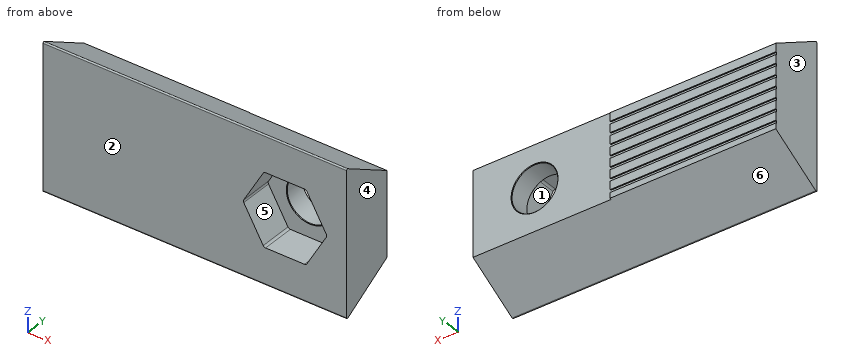
from build123d import *

# Parameters (mm, degrees)
SKETCH1_R                       = 4.15
BOSS_EXTRUDE1_DEPTH             = 10
CUT_EXTRUDE2_DEPTH              = 42.907636536
CUT_EXTRUDE2_DEPTH_BACK         = 42.907636536
SKETCH2_W                       = 0.5
SKETCH2_H                       = 0.2
BOSS_EXTRUDE2_REACH             = 43.908
BOSS_EXTRUDE2_DIRECTION_2_REACH = 43.908
SKETCH10_W                      = 15.230940108
SKETCH10_H                      = 0.2
CUT_EXTRUDE6_DEPTH              = 25
CUT_EXTRUDE5_DEPTH              = 6
FILLET3_R                       = 0.5
CHAMFER1_SIZE                   = 0.1


with BuildPart() as part:
    # Sketch1 → Boss-Extrude1 (new body)
    with BuildSketch(Plane(origin=(0, 0, 0), x_dir=(1, 0, 0), z_dir=(0, 1, 0))):
        Polygon((-15, -7.5), (15, -7.5), (40, -7.5), (40, 7.5), (15, 7.5), (-15, 7.5), align=None)
        with Locations(Location((28.85, 0, 0), (0, 0, 270))):
            Circle(SKETCH1_R, mode=Mode.SUBTRACT)
    extrude(amount=BOSS_EXTRUDE1_DEPTH)

    # Sketch2 → Cut-Extrude2 (cut, two sides: drawn at the far end of the back side and taken through both)
    with BuildSketch(Plane(origin=(0, 0, 0), x_dir=(0, 0, -1), z_dir=(1, 0, 0)).offset(-CUT_EXTRUDE2_DEPTH_BACK)):
        with Locations((-5.75, 9.9)):
            Rectangle(SKETCH2_W, SKETCH2_H)
        with Locations((-3.75, 9.9)):
            Rectangle(SKETCH2_W, SKETCH2_H)
        with Locations((-1.75, 9.9)):
            Rectangle(SKETCH2_W, SKETCH2_H)
        with Locations((0.25, 9.9)):
            Rectangle(SKETCH2_W, SKETCH2_H)
        with Locations((2.25, 9.9)):
            Rectangle(SKETCH2_W, SKETCH2_H)
        with Locations((4.25, 9.9)):
            Rectangle(SKETCH2_W, SKETCH2_H)
        with Locations((6.25, 9.9)):
            Rectangle(SKETCH2_W, SKETCH2_H)
    extrude(amount=CUT_EXTRUDE2_DEPTH + CUT_EXTRUDE2_DEPTH_BACK, mode=Mode.SUBTRACT)

    # Boss-Extrude2: up to this face of the body (flat: up to its plane)
    boss_extrude2_end = Plane(part.part.faces().sort_by_distance((40, 4.977026122, 0.001172137))[0])
    # Sketch3 → Boss-Extrude2 (add, up to the picked face)
    with BuildSketch(Plane(origin=(0, 0, 0), x_dir=(0, 0, -1), z_dir=(1, 0, 0)), mode=Mode.PRIVATE) as boss_extrude2_sk1:
        with BuildLine():
            Line((7.5, 10), (13.097822121, 0.304287674))
            ThreePointArc((13.097822121, 0.304287674), (13.097822121, 0.101429225), (12.92214155, 0))
            Line((12.92214155, 0), (7.5, 0))
            Line((7.5, 0), (7.5, 10))
        make_face()
    boss_extrude2_tool1 = split(extrude(boss_extrude2_sk1.sketch, amount=BOSS_EXTRUDE2_REACH, mode=Mode.PRIVATE), bisect_by=boss_extrude2_end, keep=Keep.BOTH, mode=Mode.PRIVATE)
    # Sketch3 → Boss-Extrude2 (add, up to the picked face)
    with BuildSketch(Plane(origin=(0, 0, 0), x_dir=(0, 0, -1), z_dir=(1, 0, 0)), mode=Mode.PRIVATE) as boss_extrude2_sk2:
        with BuildLine():
            Line((-7.5, 0), (-7.5, 10))
            Line((-7.5, 10), (-13.097822121, 0.304287674))
            ThreePointArc((-13.097822121, 0.304287674), (-13.097822121, 0.101429225), (-12.92214155, 0))
            Line((-12.92214155, 0), (-7.5, 0))
        make_face()
    boss_extrude2_tool2 = split(extrude(boss_extrude2_sk2.sketch, amount=BOSS_EXTRUDE2_REACH, mode=Mode.PRIVATE), bisect_by=boss_extrude2_end, keep=Keep.BOTH, mode=Mode.PRIVATE)
    add(boss_extrude2_tool1.solids().sort_by(Axis((0, 3.336518, -9.420866), (1, 0, 0)))[0])
    add(boss_extrude2_tool2.solids().sort_by(Axis((0, 3.336518, 9.420866), (1, 0, 0)))[0])

    # Boss-Extrude2 direction 2: up to this face of the body (flat: up to its plane)
    boss_extrude2_direction_2_end = Plane(part.part.faces().sort_by_distance((-15, 4.977026122, 0.001172137))[0])
    # Sketch3 → Boss-Extrude2 direction 2 (add, up to the picked face)
    with BuildSketch(Plane(origin=(0, 0, 0), x_dir=(0, 0, -1), z_dir=(1, 0, 0)), mode=Mode.PRIVATE) as boss_extrude2_direction_2_sk1:
        with BuildLine():
            Line((7.5, 10), (13.097822121, 0.304287674))
            ThreePointArc((13.097822121, 0.304287674), (13.097822121, 0.101429225), (12.92214155, 0))
            Line((12.92214155, 0), (7.5, 0))
            Line((7.5, 0), (7.5, 10))
        make_face()
    boss_extrude2_direction_2_tool1 = split(extrude(boss_extrude2_direction_2_sk1.sketch, amount=-BOSS_EXTRUDE2_DIRECTION_2_REACH, mode=Mode.PRIVATE), bisect_by=boss_extrude2_direction_2_end, keep=Keep.BOTH, mode=Mode.PRIVATE)
    # Sketch3 → Boss-Extrude2 direction 2 (add, up to the picked face)
    with BuildSketch(Plane(origin=(0, 0, 0), x_dir=(0, 0, -1), z_dir=(1, 0, 0)), mode=Mode.PRIVATE) as boss_extrude2_direction_2_sk2:
        with BuildLine():
            Line((-7.5, 0), (-7.5, 10))
            Line((-7.5, 10), (-13.097822121, 0.304287674))
            ThreePointArc((-13.097822121, 0.304287674), (-13.097822121, 0.101429225), (-12.92214155, 0))
            Line((-12.92214155, 0), (-7.5, 0))
        make_face()
    boss_extrude2_direction_2_tool2 = split(extrude(boss_extrude2_direction_2_sk2.sketch, amount=-BOSS_EXTRUDE2_DIRECTION_2_REACH, mode=Mode.PRIVATE), bisect_by=boss_extrude2_direction_2_end, keep=Keep.BOTH, mode=Mode.PRIVATE)
    add(boss_extrude2_direction_2_tool1.solids().sort_by(Axis((0, 3.336518, -9.420866), (-1, 0, 0)))[0])
    add(boss_extrude2_direction_2_tool2.solids().sort_by(Axis((0, 3.336518, 9.420866), (-1, 0, 0)))[0])

    # Sketch10 → Cut-Extrude6 (cut)
    with BuildSketch(Plane(origin=(40, 0, 0), x_dir=(0, 0, -1), z_dir=(1, 0, 0))):
        with Locations((0, 9.9)):
            Rectangle(SKETCH10_W, SKETCH10_H)
    extrude(amount=-CUT_EXTRUDE6_DEPTH, mode=Mode.SUBTRACT)

    # Sketch8 → Cut-Extrude5 (cut)
    with BuildSketch(Plane.XZ):
        Polygon((25.039488223, -6.6), (32.660511777, -6.6), (36.471023553, 0), (32.660511777, 6.6), (25.039488223, 6.6), (21.228976447, 0), align=None)
    extrude(amount=-CUT_EXTRUDE5_DEPTH, mode=Mode.SUBTRACT)

    # Fillet3
    fillet3_edges = [part.edges().sort_by_distance(p)[0] for p in [
        (25.039488223, 3, -6.6),
        (21.228976447, 3, 0),
        (25.039488223, 3, 6.6),
        (32.660511777, 3, 6.6),
        (36.471023553, 3, 0),
        (32.660511777, 3, -6.6),
    ]]
    fillet(fillet3_edges, radius=FILLET3_R)

    # Chamfer1
    chamfer1_edges = [part.edges().sort_by_distance(p)[0] for p in [
        (28.85, 9.8, -4.15),
        (28.85, 6, -4.15),
    ]]
    chamfer(chamfer1_edges, length=CHAMFER1_SIZE)


solid = part.part
Work out the finished part from the listing and answer in its coordinate system (mm). Face numbers are marked on the shaded views. A direction names the side the tool comes from. Round coordinates to 2 decimals unless told otherwise and drop trailing zeros. Write each loop counter-clockwise with the first axis right and the second up, starting at its lowest first coordinate (ties: lowest second). Pieces come first, ordered by that corner, then holes.
1) Given pin 1 Ø5 at (x, y) = (26.5, 4) entering from -Z; pin 2 Ø2 at (x, y) = (-8.5, 4.5) entering from +Z; pin 3 Ø2 at (x, y) = (0.5, 3) entering from +Z, each flat-ended and moving along its own axis, determine where each tip first touches the part or whether it passes through.
2) Straight lines are drawn through the part: line 1 (X direction, y = 7.05, z = 0); line 2 (Z direction, x = 28.85, y = 7.35); line 3 (Z direction, x = 28.85, y = 8). For each, find the intervals that lie inside material, in ascending order.
3) A tool of negligible diameter and unlimited length cuts with its end or side. For the marked faces 5 and 6, from which of +Z, -Z, +X, -X, +Y, -Y can it reach the whole face along a straight path? Write none if from no direction.
4) A cutting plane is placed at D-D (z = 9.5). Give the vertices of the cut face in (x, y).
5) A cutting plane is placed at A-A (x = 28.85). Give the vertices of the cut face in (y, z), plus the area to 3 significant figures.
6) A cutting plane is placed at B-B (y = 3.25). Give the vertices of the cut face in (x, z).
7) The mould has two halves that part along X. Classify the marked faces 1, 2, 3 and 4: pulls with the +X half, pulls with the -X half, needs draft (parallel to the pull), parting line crosses it, or undercut.
Completed:
1. pin 1: stops at z = -12.41
1. pin 2: stops at z = 11.25
1. pin 3: stops at z = 12.12
2. line 1: x = -15 to 24.7, 33 to 40
2. line 2: z = -9.03 to -4.15, 4.15 to 9.03
2. line 3: z = -8.65 to -4.15, 4.15 to 8.65
3. face 5: -Y
3. face 6: -Z, +X, -X, +Y
4. outline: (-15, 0) - (40, 0) - (40, 6.54) - (-15, 6.54) - close
5. outline: (0, -12.92) arc R0.2 ccw to (0.3, -13.1) - (9.8, -7.62) - (9.8, -4.25) - (9.7, -4.15) - (6.1, -4.15) - (6, -4.25) - (6, -6.6) - (0, -6.6) - close; (0, 6.6) - (6, 6.6) - (6, 4.25) - (6.1, 4.15) - (9.7, 4.15) - (9.8, 4.25) - (9.8, 7.62) - (0.3, 13.1) arc R0.2 ccw to (0, 12.92) - close
5. area: 93.9 mm2
6. outline: (-15, -11.4) - (40, -11.4) - (40, 11.4) - (-15, 11.4) - close; hole (21.37, -0.25) - (24.9, -6.35) arc R0.5 ccw to (25.33, -6.6) - (32.37, -6.6) arc R0.5 ccw to (32.8, -6.35) - (36.33, -0.25) arc R0.5 ccw to (36.33, 0.25) - (32.8, 6.35) arc R0.5 ccw to (32.37, 6.6) - (25.33, 6.6) arc R0.5 ccw to (24.9, 6.35) - (21.37, 0.25) arc R0.5 ccw to start
7. face 1: undercut
7. face 2: needs draft
7. face 3: pulls with the -X half
7. face 4: pulls with the +X half
